Work out the finished part from the listing and answer in its coordinate system (mm). Face numbers are marked on the shaded views. A direction names the side the tool comes from. Coordinates: 2 decimals unless noted, no trailing zeros. Order: outer loops, then holes, each group sorted by start corner. A loop starts at its lowest first (then second) coordinate and runs counter-clockwise, first axis right, second up. Notation, with made-up numbers: M -34,70.5 L -17,70.5 A9 cw -17,86.5 Z; hole C -7,-26 d11. An arc over 180 degrees is marked long. Answer in a Markdown table with one row per item. Add a question column.
Item 1: The part is cut by section B-B (y = -20). State how many separate pieces and enclosed holes the cut face has, then the cut area to 3 significant figures.
Item 2: Which of the six approach directions +Z, -Z, +X, -X, +Y, -Y give full straight-line access (tool end or side, diameter ignored) to the marked faces 3 and 4?
Item 3: The mould has two halves that part along X. Classify the marked faces 1 and 2: released by +X, released by -X, zero draft, split by the parting line, or undercut.
Item 4: Consider line 1 (Y direction, x = 50.5, z = 1.45); line 2 (X direction, y = -3.5, z = -0.7); line 3 (Y direction, x = 45.5, z = 0.7). Determine where each line is inside the solid, lowest interval first. Write a range as from..to.
Item 5: The part is cut by section C-C (x = -8). Write down the section's boundary in (y, z).
Item 6: The part is cut by section A-A (y = 14). Write down the section's boundary in (x, z).
Item 7: A flat-ended cylindrical pin translates along its axis: pin 1 Ø1.5 at (x, z) = (12, 0.5) entering from +Y. Find the tip coordinate at first contact, or state that the pin passes through.
from build123d import *

# Parameters (mm, degrees)
SKETCH1_R           = 1.75
BOSS_EXTRUDE1_DEPTH = 2
SCALE1_DEPTH        = 2
SCALE1_START        = -0.999756802
SCALE1_2_OUTLINE_R  = 3.5
SCALE1_2_DEPTH      = 4
FILLET1_R           = 12
FILLET3_R           = 11
FILLET5_R           = 10


# Read off the part's stored shape, not the designer's step: Scale1
with BuildPart() as part:
    # Sketch1 → Boss-Extrude1 (new body)
    with BuildSketch(Plane.XY):
        with BuildLine():
            Line((37.774530777, -2.80976251), (28.469572838, -9.10701388))
            Line((28.469572838, -9.10701388), (1.412522165, 4.616654706))
            ThreePointArc((1.412522165, 4.616654706), (-2.864052097, 1.077136302), (2.666294703, 0.594909982))
            Line((2.666294703, 0.594909982), (28.469572838, -12.71263256))
            Line((28.469572838, -12.71263256), (29.76626198, -20.464203372))
            Line((29.76626198, -20.464203372), (35.819506235, -24.004020415))
            add(Edge.make_bspline(
                [(37.774530777, -2.80976251), (45.596954448, 2.484164502), (45.142122532, -21.709783765), (35.819506235, -24.004020415)],
                knots=[0, 0, 0, 0, 1, 1, 1, 1], degree=3))
        make_face()
        with Locations((0, 1.97)):
            Circle(SKETCH1_R, mode=Mode.SUBTRACT)
        with Locations((40, -13.83)):
            Circle(SKETCH1_R, mode=Mode.SUBTRACT)
        with BuildLine():
            ThreePointArc((40, -7.58), (41.75, -5.83), (40, -4.08))
            ThreePointArc((40, -4.08), (30.675422402, -10.981359514), (34.551308869, -21.91543536))
            ThreePointArc((34.551308869, -21.91543536), (36.98051106, -21.442173575), (36.507249275, -19.012971384))
            ThreePointArc((36.507249275, -19.012971384), (34.022706668, -12.003948406), (40, -7.58))
        make_face(mode=Mode.SUBTRACT)
    extrude(amount=BOSS_EXTRUDE1_DEPTH)

    # Scale1 outline → Scale1 (cut)
    with BuildSketch(Plane.XY):
        with BuildLine():
            Line((37.166911335, -4.500685523), (40.588309586, -2.185209734))
            add(Edge.make_bspline(
                [(37.774530777, -2.80976251), (38.877601708, -2.063244904), (39.816079935, -1.903091828), (40.588309586, -2.185209734)],
                knots=[0, 0, 0, 0, 0.141013959, 0.141013959, 0.141013959, 0.141013959], degree=3))
            Line((37.774530777, -2.80976251), (29.220510655, -8.598806941))
            Line((29.220510655, -8.598806941), (30.301368209, -9.147031174))
            Line((30.301368209, -9.147031174), (32.392388987, -7.731905652))
            ThreePointArc((32.392388987, -7.731905652), (34.535363844, -5.75533272), (37.166911335, -4.500685523))
        make_face()
        with BuildLine():
            add(Edge.make_bspline(
                [(41.674674498, -2.9836722), (42.973808679, -4.53190383), (43.478218434, -7.820529427), (43.170733001, -11.35535593)],
                knots=[0.215661709, 0.215661709, 0.215661709, 0.215661709, 0.523164808, 0.523164808, 0.523164808, 0.523164808], degree=3))
            ThreePointArc((41.674674498, -2.9836722), (40.978551915, -3.529979081), (40.307930669, -4.107304814))
            ThreePointArc((40.307930669, -4.107304814), (41.743160431, -5.984569442), (40, -7.58))
            ThreePointArc((40, -7.58), (38.251209419, -7.829647385), (36.642124757, -8.558645918))
            ThreePointArc((36.642124757, -8.558645918), (34.994244779, -12.045683869), (34.064898938, -15.788845421))
            ThreePointArc((34.064898938, -15.788845421), (35.018048135, -17.603944304), (36.507249275, -19.012971384))
            ThreePointArc((36.507249275, -19.012971384), (36.98051106, -21.442173575), (34.551308869, -21.91543536))
            ThreePointArc((34.551308869, -21.91543536), (34.320026917, -21.754670705), (34.093485318, -21.587292331))
            ThreePointArc((34.093485318, -21.587292331), (34.234790142, -22.386594073), (34.409236622, -23.179322749))
            Line((34.409236622, -23.179322749), (35.819506235, -24.004020415))
            add(Edge.make_bspline(
                [(40.894606009, -19.492190926), (39.678153764, -21.750341152), (37.988934356, -23.470137935), (35.819506235, -24.004020415)],
                knots=[0.767294067, 0.767294067, 0.767294067, 0.767294067, 1, 1, 1, 1], degree=3))
            ThreePointArc((40.894606009, -19.492190926), (40.948505364, -17.126843118), (41.447135601, -14.814021622))
            ThreePointArc((41.447135601, -14.814021622), (38.35159174, -13.242420041), (41.74328031, -13.983211488))
            ThreePointArc((41.74328031, -13.983211488), (42.378136793, -12.626441553), (43.170733001, -11.35535593))
        make_face()
        Polygon((29.76626198, -20.464203372), (31.120707631, -21.256256294), (30.301368209, -16.358268534), (28.964044419, -15.668569608), align=None)
        with BuildLine():
            ThreePointArc((-2.699495917, 0.661290027), (-1.375090017, -0.696294703), (0.498906862, -0.988224458))
            Line((0.498906862, -0.988224458), (-2.699495917, 0.661290027))
        make_face()
    extrude(amount=SCALE1_DEPTH, mode=Mode.SUBTRACT)

    # Scale1 2 outline → Scale1 2 (add)
    with BuildSketch(Plane.XY.offset(SCALE1_START)):
        with BuildLine():
            add(Edge.make_bspline(
                [(48.911284088, 3.447471566), (64.556131429, 14.03532559), (63.646467598, -34.352570942), (45.001235003, -38.941044242)],
                knots=[0, 0, 0, 0, 1, 1, 1, 1], degree=3))
            Line((48.911284088, 3.447471566), (30.301368209, -9.147031174))
            Line((30.301368209, -9.147031174), (-23.812733137, 18.300305999))
            ThreePointArc((-23.812733137, 18.300305999), (-32.365881661, 11.221269191), (-21.305188061, 10.256816551))
            Line((-21.305188061, 10.256816551), (30.301368209, -16.358268534))
            Line((30.301368209, -16.358268534), (32.894746493, -31.861410158))
            Line((32.894746493, -31.861410158), (45.001235003, -38.941044242))
        make_face()
        with BuildLine():
            ThreePointArc((42.464840271, -34.763874133), (34.713067338, -12.89572244), (53.362222534, 0.906996587))
            ThreePointArc((53.362222534, 0.906996587), (56.862222534, -2.593003413), (53.362222534, -6.093003413))
            ThreePointArc((53.362222534, -6.093003413), (41.40763587, -14.940900225), (46.376721083, -28.958946182))
            ThreePointArc((46.376721083, -28.958946182), (47.323244653, -33.817350564), (42.464840271, -34.763874133))
        make_face(mode=Mode.SUBTRACT)
        with Locations((53.362222534, -18.593003413)):
            Circle(SCALE1_2_OUTLINE_R, mode=Mode.SUBTRACT)
        with Locations((-26.637777466, 13.006996587)):
            Circle(SCALE1_2_OUTLINE_R, mode=Mode.SUBTRACT)
    extrude(amount=SCALE1_2_DEPTH)

    # Fillet1
    fillet1_edges = [part.edges().sort_by_distance(p)[0] for p in [
        (30.301368209, -16.358268534, 1),
    ]]
    fillet(fillet1_edges, radius=FILLET1_R)

    # Fillet3
    fillet3_edges = [part.edges().sort_by_distance(p)[0] for p in [
        (-21.305188061, 10.256816551, 1.000243198),
    ]]
    fillet(fillet3_edges, radius=FILLET3_R)

    # Fillet5
    fillet5_edges = [part.edges().sort_by_distance(p)[0] for p in [
        (45.001235003, -38.941044242, 1.000243198),
        (32.894746493, -31.861410158, 1.000243198),
    ]]
    fillet(fillet5_edges, radius=FILLET5_R)


solid = part.part
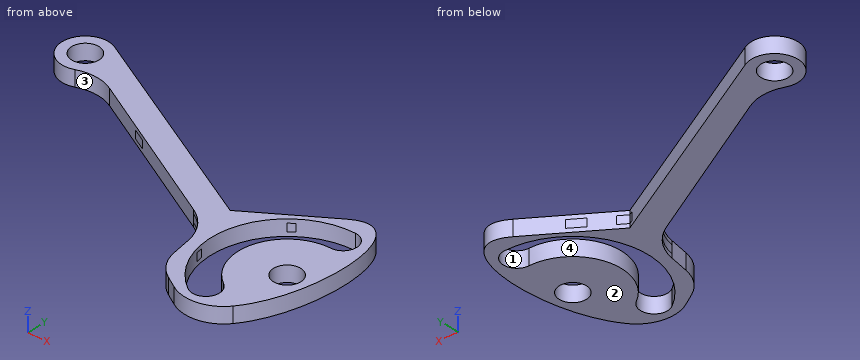
Reply:
| question | item | result |
|---|---|---|
| 1 | separate pieces | 3 |
| 1 | enclosed holes | 0 |
| 1 | area | 58.5 mm2 |
| 2 | face 3 | +Z, -Z, -Y |
| 2 | face 4 | +Z, -Z |
| 3 | face 1 | undercut |
| 3 | face 2 | zero draft |
| 4 | line 1 | y = -35.66..-20.61, -16.58..-6.43, 0.7..4.35 |
| 4 | line 2 | x = 5.37..19.17, 38.65..41.02, 56.74..59.36 |
| 4 | line 3 | y = -37.32..-35.19, -28.31..-8.88, -0.75..1.14 |
| 5 | outline | M 3.39,-1 L 10.28,-1 L 10.28,3 L 3.39,3 Z |
| 6 | outline | M -32.56,-1 L -29.99,-1 L -29.99,3 L -32.56,3 Z; M -23.28,-1 L -15.33,-1 L -15.33,3 L -23.28,3 Z |
| 7 | pin 1 | stops at y = 0.52 |
